from build123d import *

# Parameters (mm, degrees)
SKETCH1_W                 = 100
SKETCH1_H                 = 126.094412
BOSS_EXTRUDE1_DEPTH       = 5
SLOTS_DEPTH               = 11
CUT_EXTRUDE6_DEPTH        = 3
M5X0_8_TAPPED_HOLE2_D     = 4.2
SKETCH13_R                = 4.15
CUT_EXTRUDE7_DEPTH        = 5
M5X0_8_TAPPED_HOLE1_D     = 4.2
M5X0_8_TAPPED_HOLE1_DEPTH = 20
M5X0_8_TAPPED_HOLE1_TIP   = 1.2618073
CUT_EXTRUDE2_DEPTH        = 11
CUT_EXTRUDE3_DEPTH        = 11
FILLET1_R                 = 4
CHAMFER1_SIZE             = 2


with BuildPart() as part:
    # Sketch1 → Boss-Extrude1 (new body, symmetric)
    with BuildSketch(Plane(origin=(0, 0, 0), x_dir=(1, 0, 0), z_dir=(0, 1, 0))):
        with Locations((10, -5.047206)):
            Rectangle(SKETCH1_W, SKETCH1_H)
    extrude(amount=BOSS_EXTRUDE1_DEPTH, both=True)

    # Sketch3 → Slots (cut, through all)
    with BuildSketch(Plane(origin=(0, 5, 0), x_dir=(1, 0, 0), z_dir=(0, 1, 0))):
        with BuildLine():
            Line((-8.05, 0), (-8.05, -34.641016151))
            ThreePointArc((-8.05, -34.641016151), (0, -42.691016151), (8.05, -34.641016151))
            Line((8.05, -34.641016151), (8.05, 0))
            ThreePointArc((8.05, 0), (0, 8.05), (-8.05, 0))
        make_face()
        with BuildLine():
            Line((-11.95, 0), (-11.95, 20))
            ThreePointArc((-11.95, 20), (-8.449926035, 28.449926035), (0, 31.95))
            ThreePointArc((0, 31.95), (15.975, 27.669511651), (27.669511651, 15.975))
            ThreePointArc((27.669511651, 15.975), (38.666016151, 13.0284955), (41.612520652, 24.025))
            ThreePointArc((41.612520652, 24.025), (24.025, 41.612520652), (0, 48.05))
            ThreePointArc((0, 48.05), (-19.834345212, 39.834345212), (-28.05, 20))
            Line((-28.05, 20), (-28.05, 0))
            ThreePointArc((-28.05, 0), (-20, -8.05), (-11.95, 0))
        make_face()
    extrude(amount=-SLOTS_DEPTH, mode=Mode.SUBTRACT)

    # Sketch12 → Cut-Extrude6 (cut)
    with BuildSketch(Plane.XZ.offset(5)):
        with BuildLine():
            Line((10.15, 0), (10.15, 34.641016151))
            ThreePointArc((10.15, 34.641016151), (0, 44.791016151), (-10.15, 34.641016151))
            Line((-10.15, 34.641016151), (-10.15, 0))
            ThreePointArc((-10.15, 0), (0, -10.15), (10.15, 0))
        make_face()
    extrude(amount=-CUT_EXTRUDE6_DEPTH, mode=Mode.SUBTRACT)

    # M5x0.8 Tapped Hole2 (through all)
    with Locations(Plane(origin=(0, 5, 0), x_dir=(1, 0, 0), z_dir=(0, 1, 0))):
        with Locations((-20, -34.641016151)):
            Hole(M5X0_8_TAPPED_HOLE2_D / 2)

    # Sketch13 → Cut-Extrude7 (cut)
    with BuildSketch(Plane.XZ.offset(5)):
        with Locations((-20, 34.641016151)):
            Circle(SKETCH13_R)
    extrude(amount=-CUT_EXTRUDE7_DEPTH, mode=Mode.SUBTRACT)

    # M5x0.8 Tapped Hole1
    with Locations(Plane.XY.offset(68.094412)):
        with Locations((-15, 0), (35, 0)):
            Hole(M5X0_8_TAPPED_HOLE1_D / 2, depth=M5X0_8_TAPPED_HOLE1_DEPTH)
            with Locations((0, 0, -(M5X0_8_TAPPED_HOLE1_DEPTH + M5X0_8_TAPPED_HOLE1_TIP / 2))):  # 118° drill point
                Cone(0, M5X0_8_TAPPED_HOLE1_D / 2, M5X0_8_TAPPED_HOLE1_TIP, mode=Mode.SUBTRACT)

    # Sketch4 → Cut-Extrude2 (cut, through all)
    with BuildSketch(Plane(origin=(0, 5, 0), x_dir=(1, 0, 0), z_dir=(0, 1, 0))):
        Polygon((-40, 43), (-40, 58), (-25, 58), align=None)
    extrude(amount=-CUT_EXTRUDE2_DEPTH, mode=Mode.SUBTRACT)

    # Sketch5 → Cut-Extrude3 (cut, through all)
    with BuildSketch(Plane(origin=(0, 5, 0), x_dir=(1, 0, 0), z_dir=(0, 1, 0))):
        Polygon((25, 58), (60, 58), (60, 23), align=None)
    extrude(amount=-CUT_EXTRUDE3_DEPTH, mode=Mode.SUBTRACT)

    # Fillet1
    fillet1_edges = [part.edges().sort_by_distance(p)[0] for p in [
        (-25, 0, -58),
        (-40, 0, -43),
        (60, 0, -23),
        (25, 0, -58),
    ]]
    fillet(fillet1_edges, radius=FILLET1_R)

    # Chamfer1
    chamfer1_edges = [part.edges().sort_by_distance(p)[0] for p in [
        (42.5, 5, -40.5),
        (0, 5, -58),
        (-32.5, 5, -50.5),
        (-40, 5, 13.375633125),
        (-39.69551813, 5, -42.87387948),
        (-24.87387948, 5, -57.69551813),
        (24.87387948, 5, -57.69551813),
        (59.69551813, 5, -22.87387948),
        (60, 5, 23.375633125),
        (42.5, -5, -40.5),
        (-40, -5, 13.375633125),
        (-32.5, -5, -50.5),
        (0, -5, -58),
        (-39.69551813, -5, -42.87387948),
        (-24.87387948, -5, -57.69551813),
        (24.87387948, -5, -57.69551813),
        (59.69551813, -5, -22.87387948),
        (60, -5, 23.375633125),
    ]]
    chamfer(chamfer1_edges, length=CHAMFER1_SIZE)


solid = part.part
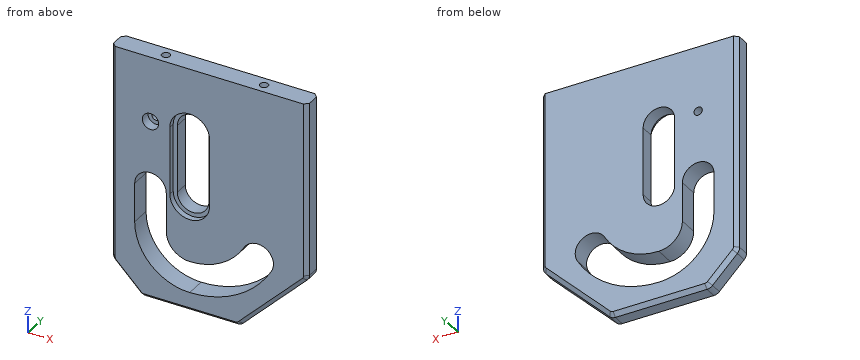
Build history of the part. All positions in model axes, mm. Give positions to 0.01 mm unless a question says otherwise; leave off trailing zeros. Loops run counter-clockwise (first coordinate to the right, second up) from the corner with the lowest first, then second, coordinate; pieces in that order, holes last. Notation, with made-up numbers: (3.5, -16) - (17.5, -16) arc R20 cw to (17.5, 13) - close; hole circle Ø11 at (83.5, 0.5). An arc over 180 degrees is marked (long way). Write item = value, one per line. Start each with the question number.
1) Band-saw the part on D-D on x = -20.5. Give the cut face in (y, z).
2) Band-saw the part on A-A on z = 50. Give the cut face in (x, y).
3) Band-saw the part on C-C on x = 15. Give the cut face in (y, z).
4) Drop flat-ended pins along their axis: pin 1 Ø4 at (x, z) = (-20, 34.64) entering from -Y; pin 2 Ø2 at (x, y) = (38, -2.5) entering from -Z; pin 3 Ø6 at (y, z) = (0, -44) entering from +X; pin 4 Ø3.5 at (x, y) = (-15, 0) entering from +Z. Give the stop position or say it passes through.
5) Probe probe 1 along X at (y, z) = (0, 61.75); probe 2 along X at (y, z) = (4, -25.5); probe 3 along Y at (x, z) = (35, 60.5). List the from-to ranges inside material, lowest first. Write a range as from..to.
6) Band-saw the part on B-B on x = 3.5. Give the cut face in (y, z).
Final values:
q1.outline = (-5, -56) - (-3, -58) - (3, -58) - (5, -56) - (5, -39.15) - (-5, -39.15) - close; (-5, 8.03) - (5, 8.03) - (5, 32.6) - (0, 32.6) - (0, 30.52) - (-5, 30.52) - close; (-5, 38.76) - (0, 38.76) - (0, 36.68) - (5, 36.68) - (5, 68.09) - (-5, 68.09) - close
q2.outline = (-40, -3) - (-38, -5) - (58, -5) - (60, -3) - (60, 3) - (58, 5) - (-38, 5) - (-40, 3) - close; hole circle Ø4.2 at (-15, 0); hole circle Ø4.2 at (35, 0)
q3.outline = (-5, -56) - (-3, -58) - (3, -58) - (5, -56) - (5, -45.65) - (-5, -45.65) - close; (-5, -28.21) - (5, -28.21) - (5, 68.09) - (-5, 68.09) - close
q4.pin_1 = through
q4.pin_2 = -46
q4.pin_3 = 42
q4.pin_4 = 47.88
q5.probe_1 = -40..-17.1, -12.9..32.9, 37.1..60
q5.probe_2 = -39..-27.51, -10.61..19.25, 40.73..56.09
q5.probe_3 = -5..-2.1, 2.1..5
q6.outline = (-5, -56) - (-3, -58) - (3, -58) - (5, -56) - (5, -47.92) - (-5, -47.92) - close; (-5, -31.76) - (5, -31.76) - (5, -7.25) - (-2, -7.25) - (-2, -9.53) - (-5, -9.53) - close; (-5, 44.17) - (-2, 44.17) - (-2, 41.89) - (5, 41.89) - (5, 68.09) - (-5, 68.09) - close
